Check sheet for the modelled part. Datum: model origin and axes. Units: mm. A direction names the side the tool comes from. Give positions to 0.01 mm unless a question says otherwise; leave off trailing zeros. Loops run counter-clockwise (first coordinate to the right, second up) from the corner with the lowest first, then second, coordinate; pieces in that order, holes last.
```python
from build123d import *

# Parameters (mm, degrees)
SKETCH_W        = 70
SKETCH_H        = 70
PAD_DEPTH       = 70
SKETCH001_W     = 60
SKETCH001_H     = 60
POCKET_DEPTH    = 65
SKETCH002_W     = 65
SKETCH002_H     = 65
POCKET001_DEPTH = 2.5
SKETCH004_W     = 12.5
SKETCH004_H     = 12.5
PAD001_DEPTH    = 8
SKETCH005_R     = 1.375
POCKET002_DEPTH = 10
SKETCH006_R     = 14
POCKET003_DEPTH = 70.001
FILLET_R        = 5
FILLET001_R     = 5
FILLET002_R     = 5
CHAMFER_SIZE    = 1.5


with BuildPart() as part:
    # Sketch → Pad (new body)
    with BuildSketch(Plane.XY):
        Rectangle(SKETCH_W, SKETCH_H)
    extrude(amount=PAD_DEPTH)

    # Sketch001 → Pocket (cut)
    with BuildSketch(Plane.XY):
        Rectangle(SKETCH001_W, SKETCH001_H)
    extrude(amount=POCKET_DEPTH, mode=Mode.SUBTRACT)

    # Sketch002 → Pocket001 (cut)
    with BuildSketch(Plane.XY):
        Rectangle(SKETCH002_W, SKETCH002_H)
    extrude(amount=POCKET001_DEPTH, mode=Mode.SUBTRACT)

    # Sketch004 (on DatumPlane) → Pad001 (join)
    with BuildSketch(Plane.XY.offset(7)):
        with Locations((-23.75, 23.75)):
            Rectangle(SKETCH004_W, SKETCH004_H)
        with Locations((23.75, 23.75)):
            Rectangle(SKETCH004_W, SKETCH004_H)
        with Locations((-23.75, -23.75)):
            Rectangle(SKETCH004_W, SKETCH004_H)
        with Locations((23.75, -23.75)):
            Rectangle(SKETCH004_W, SKETCH004_H)
    extrude(amount=PAD001_DEPTH)

    # Sketch005 (on DatumPlane) → Pocket002 (cut)
    with BuildSketch(Plane.XY.offset(7)):
        with Locations((-22.5, 22.5)):
            Circle(SKETCH005_R)
        with Locations((22.5, 22.5)):
            Circle(SKETCH005_R)
        with Locations((22.5, -22.5)):
            Circle(SKETCH005_R)
        with Locations((-22.5, -22.5)):
            Circle(SKETCH005_R)
    extrude(amount=POCKET002_DEPTH, mode=Mode.SUBTRACT)

    # Sketch006 → Pocket003 (cut, through all)
    with BuildSketch(Plane.XY):
        Circle(SKETCH006_R)
    extrude(amount=POCKET003_DEPTH, mode=Mode.SUBTRACT)

    # Fillet
    fillet_edges = [part.edges().sort_by_distance(p)[0] for p in [
        (17.5, 30, 11),
        (17.5, 17.5, 11),
        (30, 17.5, 11),
        (30, -17.5, 11),
        (17.5, -17.5, 11),
        (17.5, -30, 11),
        (-17.5, -30, 11),
        (-17.5, -17.5, 11),
        (-30, -17.5, 11),
        (-30, 17.5, 11),
        (-17.5, 17.5, 11),
        (-17.5, 30, 11),
    ]]
    fillet(fillet_edges, radius=FILLET_R)

    # Fillet001
    fillet001_edges = [part.edges().sort_by_distance(p)[0] for p in [
        (30, 30, 4.75),
        (30, -30, 4.75),
        (-30, -30, 4.75),
        (-30, 30, 4.75),
    ]]
    fillet(fillet001_edges, radius=FILLET001_R)

    # Fillet002
    fillet002_edges = [part.edges().sort_by_distance(p)[0] for p in [
        (32.5, -32.5, 1.25),
        (32.5, 32.5, 1.25),
        (-32.5, 32.5, 1.25),
        (-32.5, -32.5, 1.25),
    ]]
    fillet(fillet002_edges, radius=FILLET002_R)

    # Chamfer
    chamfer_edges = [part.edges().sort_by_distance(p)[0] for p in [
        (35, 35, 35),
        (0, 35, 0),
        (35, 0, 0),
        (-35, 35, 35),
        (0, 35, 70),
        (-35, 0, 70),
        (0, -35, 70),
        (35, 0, 70),
        (-35, -35, 35),
        (-35, 0, 0),
        (0, -35, 0),
        (35, -35, 35),
    ]]
    chamfer(chamfer_edges, length=CHAMFER_SIZE)


solid = part.part
```
(1) Gauge pin test, flat ends, axial feed: pin 1 Ø19 at (x, y) = (19.5, 21) entering from -Z; pin 2 Ø19 at (x, y) = (-17.5, -25) entering from -Z; pin 3 Ø5 at (x, y) = (-22.5, 23.5) entering from -Z; pin 4 Ø5 at (x, y) = (-8.5, 11.5) entering from -Z. Record the tip position at first contact, or that the pin passes through.
(2) Release check for a two-part mould opening along Y. For faces 1 (the face through (0, -30, 33)), 2 (the face through (-15, 0, 70)), 3 (the face through (31, 31.07, 1.27)) record: pulls with the +Y half, pulls with the -Y half, needs draft (parallel to the pull), parting line crosses it, or undercut.
(3) Section check B-B on z = 57.5. Record the boundary of the cut face in (x, y).
(4) Section check D-D on x = -19. Record the boundary of the cut face in (y, z).
(5) Section check C-C on x = -10. Record the boundary of the cut face in (y, z).
(6) Access from +Z, -Z, +X, -X, +Y, -Y to the whole of each face (thin tool, end or side, straight path). Record for faces 4 (the face through (-17.5, 24, 11)), 5 (the face through (-23, 25, 15)), 6 (the face through (12.932, -5.362, 67.465)).
(7) Section check A-A on y = 0. Record the boundary of the cut face in (x, z).
(8) Material ranges on line 1 (X direction, y = -22.5, z = 11.5) (3 decimals); line 2 (X direction, y = 19.5, z = 45), recorded low to high.
Computed values:
1. pin 1: stops at z = 2.5
1. pin 2: stops at z = 0
1. pin 3: stops at z = 7
1. pin 4: stops at z = 65
2. face 1: undercut
2. face 2: needs draft
2. face 3: undercut
3. outline: (-35, -33.5) - (-33.5, -35) - (33.5, -35) - (35, -33.5) - (35, 33.5) - (33.5, 35) - (-33.5, 35) - (-35, 33.5) - close; hole (-30, -30) - (30, -30) - (30, 30) - (-30, 30) - close
4. outline: (-35, 1.5) - (-33.5, 0) - (-32.5, 0) - (-32.5, 2.5) - (-30, 2.5) - (-30, 7) - (-18.93, 7) - (-18.93, 15) - (-30, 15) - (-30, 65) - (30, 65) - (30, 15) - (18.93, 15) - (18.93, 7) - (30, 7) - (30, 2.5) - (32.5, 2.5) - (32.5, 0) - (33.5, 0) - (35, 1.5) - (35, 68.5) - (33.5, 70) - (-33.5, 70) - (-35, 68.5) - close
5. outline: (-35, 1.5) - (-33.5, 0) - (-32.5, 0) - (-32.5, 2.5) - (-30, 2.5) - (-30, 65) - (-9.8, 65) - (-9.8, 70) - (-33.5, 70) - (-35, 68.5) - close; (9.8, 65) - (30, 65) - (30, 2.5) - (32.5, 2.5) - (32.5, 0) - (33.5, 0) - (35, 1.5) - (35, 68.5) - (33.5, 70) - (9.8, 70) - close
6. face 4: -Z
6. face 5: none
6. face 6: +Z, -Z
7. outline: (-35, 1.5) - (-33.5, 0) - (-32.5, 0) - (-32.5, 2.5) - (-30, 2.5) - (-30, 65) - (-14, 65) - (-14, 70) - (-33.5, 70) - (-35, 68.5) - close; (14, 65) - (30, 65) - (30, 2.5) - (32.5, 2.5) - (32.5, 0) - (33.5, 0) - (35, 1.5) - (35, 68.5) - (33.5, 70) - (14, 70) - close
8. line 1: x = -35 to -23.875, -21.125 to -17.5, 17.5 to 21.125, 23.875 to 35
8. line 2: x = -35 to -30, 30 to 35
